Can you work these out from the drawing? Everything is in mm from the part's minimum corner. A direction names the side the tool comes from. Give positions to 0.01 mm unless a question says otherwise; leave off trailing zeros. Order: outer loops, then holes, each group sorted by start corner. A loop starts at its lowest first (then second) coordinate and runs counter-clockwise, first axis right, second up. Notation, with made-up numbers: (0, 48.25) -> (48, 48.25) arc R12 cw to (48, 54.25) -> close; hole circle Ø10 at (72.25, 41). An arc over 180 degrees is marked (long way). One line per item, written item: value.
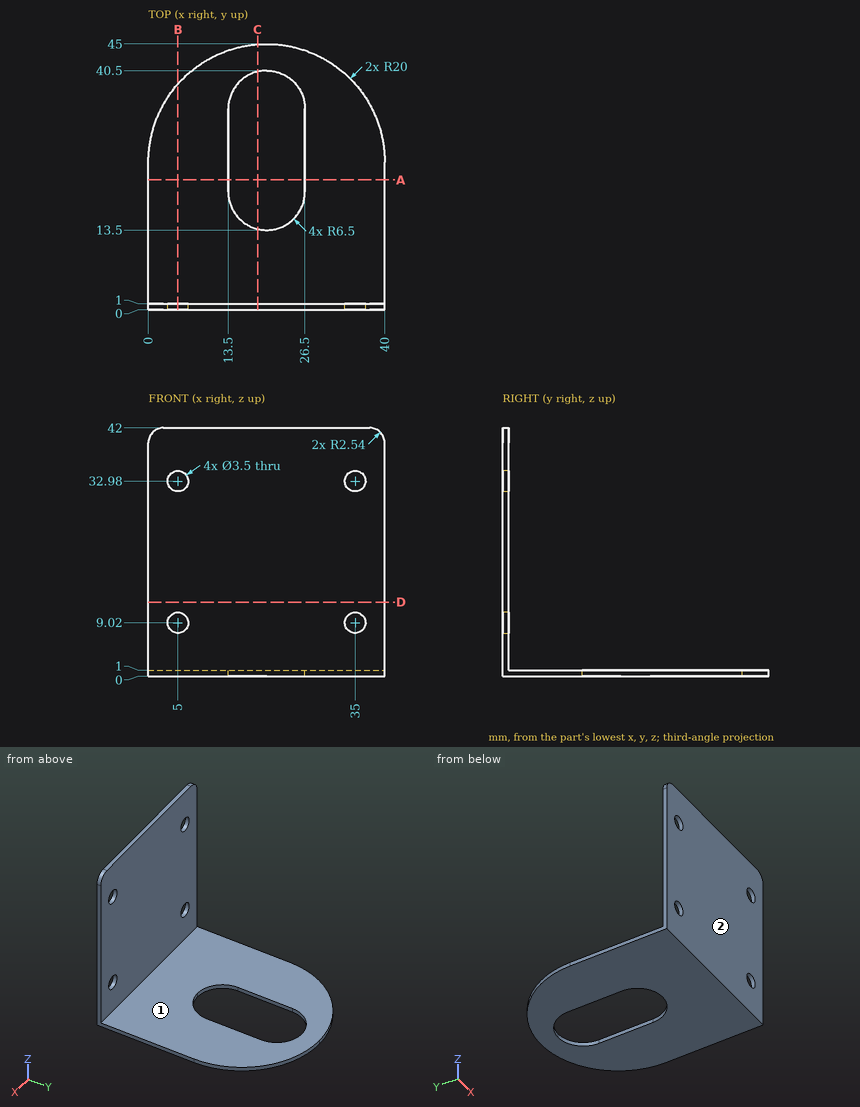
1) For the marked faces 1 and 2, which set-ups out of +Z, -Z, +X, -X, +Y, -Y let a thin tool reach every point of the face, with its end or its side?
Answer below:
face 1: +Z, +X, -X, +Y
face 2: +Z, -Z, +X, -X, -Y
2) Suppose I cut it at A-A, the plane y = 22. Write out the boundary of the cut face in (x, z).
Answer below:
outline: (0, 0) -> (13.5, 0) -> (13.5, 1) -> (0, 1) -> close; (26.5, 0) -> (40, 0) -> (40, 1) -> (26.5, 1) -> close
3) For P1, Ø0.8, axis at y = 29.5, z = 0.5, coming from the +X side (1 decimal); P2, Ø3, axis at x = 35, z = 32.98, coming from the -Y side; P3, Ø8, axis at x = 16.5, z = 26, coming from the -Y side; P4, Ø12, axis at x = 11, z = 24, coming from the +Y side, each with a flat end and sliding along its axis, tell me the tip position at first contact or that it passes through.
Answer below:
P1: stops at x = 39.6
P2: passes through
P3: stops at y = 0
P4: stops at y = 1
4) Suppose I cut it at D-D, the plane z = 12.5. Write out the boundary of the cut face in (x, y).
Answer below:
outline: (0, 0) -> (40, 0) -> (40, 1) -> (0, 1) -> close
5) If I drill on line 1 along Y through (x, z) = (25, 38.5), over which ranges is the centre line in solid material (lowest first)?
Answer below:
line 1: y = 0 to 1
6) Suppose I cut it at B-B, the plane x = 5. Write out the boundary of the cut face in (y, z).
Answer below:
outline: (0, 0) -> (38.23, 0) -> (38.23, 1) -> (1, 1) -> (1, 7.27) -> (0, 7.27) -> close; (0, 10.77) -> (1, 10.77) -> (1, 31.23) -> (0, 31.23) -> close; (0, 34.73) -> (1, 34.73) -> (1, 42) -> (0, 42) -> close
7) Suppose I cut it at C-C, the plane x = 18.5. Write out the boundary of the cut face in (y, z) (1 decimal).
Answer below:
outline: (0, 0) -> (13.7, 0) -> (13.7, 1) -> (1, 1) -> (1, 42) -> (0, 42) -> close; (40.3, 0) -> (44.9, 0) -> (44.9, 1) -> (40.3, 1) -> close
